The listing builds one solid part. Answer for the finished solid, in the listing's coordinates (mm). A direction names the side the tool comes from. Round coordinates to 2 decimals unless told otherwise and drop trailing zeros. Write each loop counter-clockwise with the first axis right and the second up, starting at its lowest first coordinate (ties: lowest second). Pieces come first, ordered by that corner, then holes.
Item 1: Find section D-D on x = -94. Give the vertices of the cut face in (y, z).
Item 2: For a pull along Y with two mould halves and no side action, classify faces 6 (the face through (-7.518, 7.129, 30.42)), 7 (the face through (0, 143, 30)), 8 (the face through (-30.488, 33.718, 29.58)) as +Y half, -Y half, draft (parallel to the pull), parting line (faces both ways), or undercut.
Item 3: Find section B-B on y = 205.5. Give the vertices of the cut face in (x, z), then the cut area to 3 significant figures.
Item 4: Find the intervals of material crossed by probe 1 along Y at (x, z) = (-30, 44); probe 2 along X at (y, z) = (30, 17.5); probe 3 along Y at (x, z) = (-144, 48), in increasing order.
Item 5: Find section A-A on y = 30. Give the vertices of the cut face in (x, z).
Item 6: Each of these flat-tipped pins is pushed along its axis until it touches: pin 1 (12 mm diameter, centred on x = -30, y = 30, fed in from -Z); pin 2 (5 mm diameter, centred on y = 87.5, z = 118.5, fed in from +X); pin 3 (1 mm diameter, centred on y = 114, z = 131.5, fed in from -X); pin 4 (8 mm diameter, centred on y = 148.5, z = 87.5, fed in from +X). Where does it stop, or does it pass through?
Item 7: A tool of negligible diameter and unlimited length cuts with its end or side. For faces 1 (the face through (-87.724, 146.47, 70.168)), 2 (the face through (-135, 144, 80)), 3 (the face through (-88, 40, 94)), 4 (the face through (-88, 250, 94)), 5 (the face through (-40, 144, 80)), from which of +Z, -Z, +X, -X, +Y, -Y can it reach the whole face along a straight path? Write none if from no direction.
Item 8: Find section C-C on x = -145. Give the vertices of the cut face in (y, z).
```python
from build123d import *

# Parameters (mm, degrees)
IZIM4_W                     = 175
IZIM4_H                     = 290
Y_KSEKLIK_EKSTR_ZYON5_DEPTH = 60
RADYUS4_R                   = 25
KES_EKSTR_ZYON2_DEPTH       = 344.984011256
KES_EKSTR_ZYON2_DEPTH_BACK  = 344.984011256
IZIM8_R                     = 3.75
IZIM9_W                     = 95
IZIM9_H                     = 210
Y_KSEKLIK_EKSTR_ZYON8_DEPTH = 90
KES_EKSTR_ZYON4_DEPTH       = 341.036762718
KES_EKSTR_ZYON8_DEPTH       = 341.036762718


with BuildPart() as part:
    # Çizim4 → Yükseklik-Ekstrüzyon5 (new body)
    with BuildSketch(Plane.XY):
        with Locations((-87.5, 145)):
            Rectangle(IZIM4_W, IZIM4_H)
    extrude(amount=Y_KSEKLIK_EKSTR_ZYON5_DEPTH)

    # Radyus4
    radyus4_edges = [part.edges().sort_by_distance(p)[0] for p in [
        (0, 0, 30),
        (-175, 0, 30),
        (-175, 290, 30),
        (0, 290, 30),
    ]]
    fillet(radyus4_edges, radius=RADYUS4_R)

    # Çizim8 → Kes-Ekstrüzyon2 (cut, two sides: drawn at the far end of the back side and taken through both)
    with BuildSketch(Plane.XY.offset(60).offset(-KES_EKSTR_ZYON2_DEPTH_BACK)):
        with Locations((-145, 30)):
            Circle(IZIM8_R)
        with Locations((-30, 30)):
            Circle(IZIM8_R)
        with Locations((-145, 260)):
            Circle(IZIM8_R)
        with Locations((-30, 260)):
            Circle(IZIM8_R)
    extrude(amount=KES_EKSTR_ZYON2_DEPTH + KES_EKSTR_ZYON2_DEPTH_BACK, mode=Mode.SUBTRACT)

    # Çizim9 → Yükseklik-Ekstrüzyon8 (add)
    with BuildSketch(Plane.XY.offset(60)):
        with Locations((-87.5, 145)):
            Rectangle(IZIM9_W, IZIM9_H)
    extrude(amount=Y_KSEKLIK_EKSTR_ZYON8_DEPTH)

    # Çizim11 → Kes-Ekstrüzyon4 (cut, through all)
    with BuildSketch(Plane(origin=(0, 250, 0), x_dir=(1, 0, 0), z_dir=(0, 1, 0))):
        Polygon((-40, -100), (-87.5, -150), (-40, -150), align=None)
        Polygon((-87.5, -150), (-135, -100), (-135, -150), align=None)
    extrude(amount=-KES_EKSTR_ZYON4_DEPTH, mode=Mode.SUBTRACT)

    # Çizim16 → Kes-Ekstrüzyon8 (cut, through all)
    with BuildSketch(Plane(origin=(0, 250, 0), x_dir=(1, 0, 0), z_dir=(0, 1, 0))):
        with BuildLine():
            Line((-77.329660293, -60), (-97.670339707, -60))
            ThreePointArc((-97.670339707, -60), (-87.5, -70.170339707), (-77.329660293, -60))
        make_face()
    extrude(amount=-KES_EKSTR_ZYON8_DEPTH, mode=Mode.SUBTRACT)


solid = part.part
```
Check values:
1. outline: (0, 0) - (290, 0) - (290, 60) - (0, 60) - close; (40, 67.82) - (250, 67.82) - (250, 143.16) - (40, 143.16) - close
2. face 6: -Y half
2. face 7: draft
2. face 8: undercut
3. outline: (-175, 0) - (0, 0) - (0, 60) - (-40, 60) - (-40, 100) - (-87.5, 150) - (-135, 100) - (-135, 60) - (-175, 60) - close; hole (-97.67, 60) - (-77.33, 60) arc R10.17 ccw to start
3. area: 16,500 mm2
4. probe 1: y = 0 to 26.25, 33.75 to 256.25, 263.75 to 290
4. probe 2: x = -175 to -148.75, -141.25 to -33.75, -26.25 to 0
4. probe 3: y = 0 to 26.39, 33.61 to 256.39, 263.61 to 290
5. outline: (-175, 0) - (-148.75, 0) - (-148.75, 60) - (-175, 60) - close; (-141.25, 0) - (-33.75, 0) - (-33.75, 60) - (-141.25, 60) - close; (-26.25, 0) - (0, 0) - (0, 60) - (-26.25, 60) - close
6. pin 1: stops at z = 0
6. pin 2: stops at x = -55.2
6. pin 3: stops at x = -105.55
6. pin 4: stops at x = -40
7. face 1: +Y, -Y
7. face 2: +Z, -X, +Y, -Y
7. face 3: +Z, +X, -X, -Y
7. face 4: +Z, +X, -X, +Y
7. face 5: +Z, +X, +Y, -Y
8. outline: (0, 0) - (26.25, 0) - (26.25, 60) - (0, 60) - close; (33.75, 0) - (256.25, 0) - (256.25, 60) - (33.75, 60) - close; (263.75, 0) - (290, 0) - (290, 60) - (263.75, 60) - close
